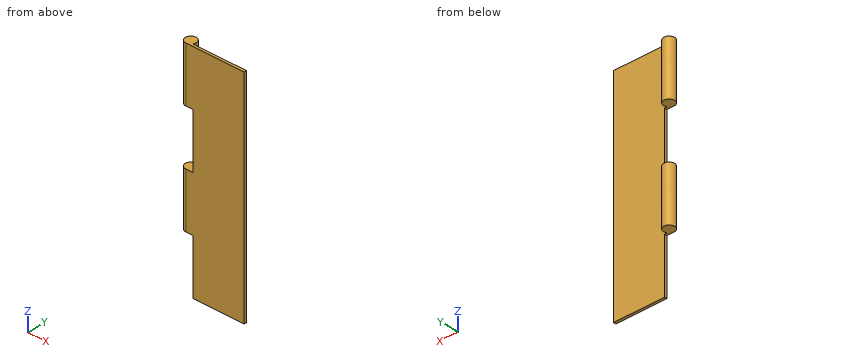
from build123d import *

# Parameters (mm, degrees)
EXTRUSION1_DEPTH           = 60
EXTRUSION2_START           = -10
ESQUISSE2_W                = 7.046962448
ESQUISSE2_H                = 15
EXTRUSION2_DEPTH           = 73.139279043
R_P_TITION_LIN_AIRE1_COUNT = 2
R_P_TITION_LIN_AIRE1_PITCH = 30


with BuildPart() as part:
    # Esquisse1 → Extrusion1 (new body)
    with BuildSketch(Plane.XY):
        with BuildLine():
            Line((0, 0), (16, 0))
            Line((16, 0), (16, 0.7))
            Line((16, 0.7), (1.268857754, 0.7))
            ThreePointArc((1.268857754, 0.7), (-0.724568837, 2.813392554), (0, 0))
        make_face()
    extrude(amount=EXTRUSION1_DEPTH)

    # Esquisse2 → Extrusion2 (cut, through all)
    with BuildSketch(Plane(origin=(0, 0.7, 0), x_dir=(1, 0, 0), z_dir=(0, 1, 0)).offset(EXTRUSION2_START)):
        with Locations((-1.523481224, -37.5)):
            Rectangle(ESQUISSE2_W, ESQUISSE2_H)
    extrusion2 = extrude(amount=EXTRUSION2_DEPTH, mode=Mode.SUBTRACT)

    # Répétition linéaire1: Extrusion2 ×2
    with Locations(*[(0, 0, -i * R_P_TITION_LIN_AIRE1_PITCH) for i in range(1, R_P_TITION_LIN_AIRE1_COUNT)]):
        add(extrusion2, mode=Mode.SUBTRACT)


solid = part.part
CAD build for the part. Positions are in the model's coordinates, mm. Round coordinates to 2 decimals unless told otherwise and drop trailing zeros. Loops run counter-clockwise (first coordinate to the right, second up) from the corner with the lowest first, then second, coordinate; pieces in that order, holes last. Notation, with made-up numbers: (69, 50) - (103, 50) arc R12 cw to (103, 57) - close; hole circle Ø1 at (39.25, 85). An arc over 180 degrees is marked (long way). Put each result on its own line as item: value.
1. Slice it at A-A on y = 1.5. List the corners of the cut face in (x, z), and give its area (3 significant figures).
Geometry check:
outline: (-1.5, 15) - (1.5, 15) - (1.5, 30) - (-1.5, 30) - close; (-1.5, 45) - (1.5, 45) - (1.5, 60) - (-1.5, 60) - close
area: 90.0 mm²
2. Slice it at B-B on z = 25. List the corners of the cut face in (x, y).
Geometry check:
outline: (0, 0) - (16, 0) - (16, 0.7) - (1.27, 0.7) arc R1.5 ccw (long way) to start
3. Pin check, flat tips, straight feed: P1, Ø4.5, axis at x = 8, z = 27, coming from the +Y side; P2, Ø0.6, axis at y = 0, z = 39, coming from the -X side. Stop position of each tip, or through.
Geometry check:
P1: y = 0.7
P2: x = 2
4. Slice it at C-C on x = 4. List the corners of the cut face in (y, z).
Geometry check:
outline: (0, 0) - (0.7, 0) - (0.7, 60) - (0, 60) - close
5. Wall check: line 1 (Z direction, x = 0, y = 1.85); line 2 (Y direction, x = 8.25, z = 25); line 3 (X direction, y = 0.6, z = 3.5). Give the ranges that are in metal, low to high.
Geometry check:
line 1: 15 to 30, 45 to 60
line 2: 0 to 0.7
line 3: 2 to 16
